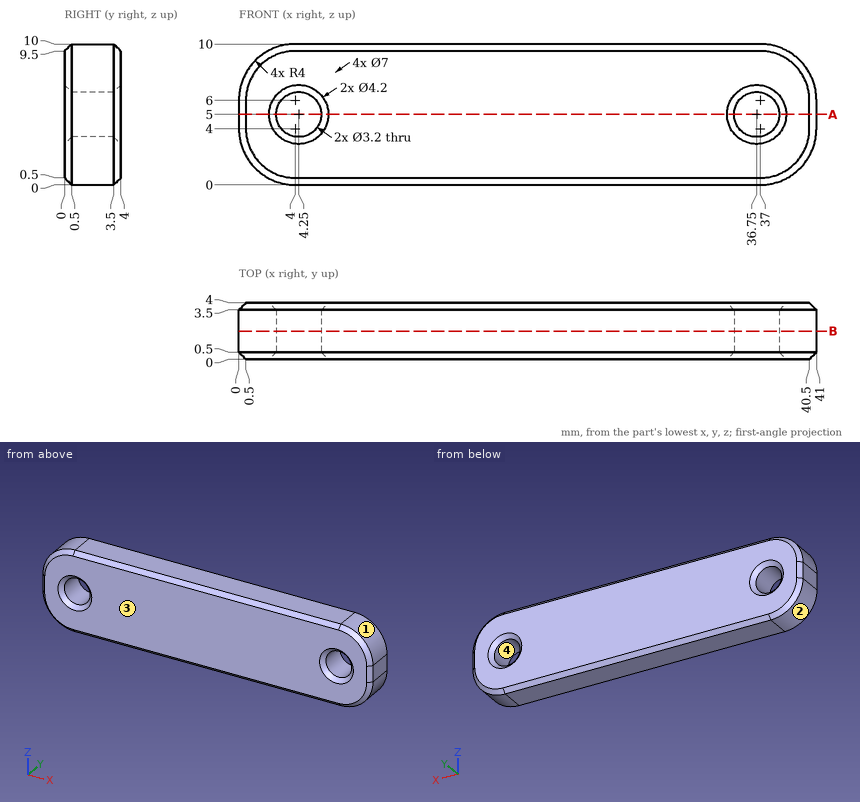
Here's the drawing with two shaded views (mm, measured from the low corner). I have some questions. Coordinates: 2 decimals unless noted, no trailing zeros. Loops run counter-clockwise (first coordinate to the right, second up) from the corner with the lowest first, then second, coordinate; pieces in that order, holes last.
Item 1: Suppose I cut it at A-A (z = 5). Please give me the cut outline in (x, y).
Answers below:
outline: (0, 0.5) - (0.5, 0) - (2.15, 0) - (2.65, 0.5) - (2.65, 3.5) - (2.15, 4) - (0.5, 4) - (0, 3.5) - close; (5.85, 0.5) - (6.35, 0) - (34.65, 0) - (35.15, 0.5) - (35.15, 3.5) - (34.65, 4) - (6.35, 4) - (5.85, 3.5) - close; (38.35, 0.5) - (38.85, 0) - (40.5, 0) - (41, 0.5) - (41, 3.5) - (40.5, 4) - (38.85, 4) - (38.35, 3.5) - close
Item 2: Please list where these lines run through material, in increasing order: L1, parallel to X at y = 2.1, z = 5; L2, parallel to X at y = 1.75, z = 6.25; L3, parallel to Z at x = 4.5, y = 0.2.
Answers below:
L1: x = 0 to 2.65, 5.85 to 35.15, 38.35 to 41
L2: x = 0.01 to 3.25, 5.25 to 35.75, 37.75 to 40.99
L3: z = 0.3 to 3.12, 6.88 to 9.7
Item 3: If we mould it in two halves opening along Z, with no side actions, what happens to the marked faces 1, 2, 3 and 4? For each: released by +Z, released by -Z, zero draft, split by the parting line, or undercut.
Answers below:
face 1: released by +Z
face 2: released by -Z
face 3: zero draft
face 4: undercut
Item 4: Suppose I cut it at B-B (y = 2). Please give me the cut outline in (x, z), then the cut area to 3 significant figures.
Answers below:
outline: (0, 4) arc R4 ccw to (4, 0) - (37, 0) arc R4 ccw to (41, 4) - (41, 6) arc R4 ccw to (37, 10) - (4, 10) arc R4 ccw to (0, 6) - close; hole circle Ø3.2 at (4.25, 5); hole circle Ø3.2 at (36.75, 5)
area: 380 mm2
Item 5: I'm going to push flat-ended pins straight in: pin 1 (2 mm diameter, centred on x = 25, z = 5, fed in from -Y); pin 2 (3.5 mm diameter, centred on x = 36.75, z = 5, fed in from +Y); pin 3 (2 mm diameter, centred on y = 2.5, z = 8, fed in from +X). Where does each tip first touch, or does it pass through?
Answers below:
pin 1: stops at y = 0
pin 2: stops at y = 3.65
pin 3: stops at x = 40.87
